Verification items for the finished model (mm, model axes). Face numbers are marked on the shaded views. A direction names the side the tool comes from. Round coordinates to 2 decimals unless told otherwise and drop trailing zeros. Loops run counter-clockwise (first coordinate to the right, second up) from the corner with the lowest first, then second, coordinate; pieces in that order, holes last. Notation, with made-up numbers: M -17.75,74.5 L -13.75,74.5 A18 cw -13.75,106.5 Z; hole C -31.75,1 d10. An arc over 180 degrees is marked long. Answer as CSV lines item,"result".
```python
from build123d import *

# Parameters (mm, degrees)
BOSS_EXTRUDE1_DEPTH = 4
BOSS_EXTRUDE2_DEPTH = 2.25
SKETCH3_R           = 7.925
CUT_EXTRUDE1_DEPTH  = 9.25
SKETCH4_R           = 2
CUT_EXTRUDE2_DEPTH  = 9.25
CUT_EXTRUDE3_DEPTH  = 3
FILLET1_R           = 2.36
CHAMFER1_SIZE       = 3.5
CHAMFER1_SIZE2      = 2.020725942
BOSS_EXTRUDE3_DEPTH = 4
FILLET2_R           = 2


with BuildPart() as part:
    # Sketch1 → Boss-Extrude1 (new body)
    with BuildSketch(Plane(origin=(0, 0, 0), x_dir=(1, 0, 0), z_dir=(0, 1, 0))):
        with BuildLine():
            Line((-13.29118379, 20.889836125), (-0.68999579, 20.889836125))
            Line((-0.68999579, 20.889836125), (-0.68999579, 24.09210312))
            Line((-0.68999579, 24.09210312), (-0.68999579, 26.09210312))
            Line((-0.68999579, 26.09210312), (12.01000421, 26.09210312))
            Line((12.01000421, 26.09210312), (12.01000421, 24.09210312))
            Line((12.01000421, 24.09210312), (12.01000421, -26.90789688))
            Line((12.01000421, -26.90789688), (12.01000421, -28.90789688))
            Line((12.01000421, -28.90789688), (-0.68999579, -28.90789688))
            Line((-0.68999579, -28.90789688), (-0.68999579, -26.90789688))
            Line((-0.68999579, -26.90789688), (-0.68999579, -23.705629885))
            Line((-0.68999579, -23.705629885), (-13.29118379, -23.705629885))
            ThreePointArc((-13.29118379, -23.705629885), (-35.588916795, -1.40789688), (-13.29118379, 20.889836125))
        make_face()
    extrude(amount=BOSS_EXTRUDE1_DEPTH)

    # Sketch2 → Boss-Extrude2 (add)
    with BuildSketch(Plane(origin=(0, 4, 0), x_dir=(1, 0, 0), z_dir=(0, 1, 0))):
        with BuildLine():
            Line((-0.68999579, 20.889836125), (-0.68999579, 16.987726462))
            ThreePointArc((-0.68999579, 16.987726462), (9.006549215, -1.40789688), (-0.68999579, -19.803520222))
            Line((-0.68999579, -19.803520222), (-0.68999579, -23.705629885))
            Line((-0.68999579, -23.705629885), (-13.29118379, -23.705629885))
            ThreePointArc((-13.29118379, -23.705629885), (-35.588916795, -1.40789688), (-13.29118379, 20.889836125))
            Line((-13.29118379, 20.889836125), (-0.68999579, 20.889836125))
        make_face()
    extrude(amount=BOSS_EXTRUDE2_DEPTH)

    # Sketch3 → Cut-Extrude1 (cut)
    with BuildSketch(Plane.XZ):
        with Locations(Location((-13.29118379, 1.40789688, 0), (0, 0, 270))):
            Circle(SKETCH3_R)
    extrude(amount=-CUT_EXTRUDE1_DEPTH, mode=Mode.SUBTRACT)

    # Sketch4 → Cut-Extrude2 (cut)
    with BuildSketch(Plane.XZ):
        with Locations(Location((3.31000421, -21.59210312, 0), (0, 0, 270))):
            Circle(SKETCH4_R)
        with Locations(Location((3.31000421, 24.40789688, 0), (0, 0, 270))):
            Circle(SKETCH4_R)
    extrude(amount=-CUT_EXTRUDE2_DEPTH, mode=Mode.SUBTRACT)

    # Sketch5 → Cut-Extrude3 (cut)
    with BuildSketch(Plane.XZ):
        with BuildLine():
            ThreePointArc((-20.901279021, -7.773174712), (-25.21618379, 1.40789688), (-20.901279021, 10.588968471))
            Line((-20.901279021, 10.588968471), (-24.18129969, 16.27013092))
            ThreePointArc((-24.18129969, 16.27013092), (-31.71618379, 1.40789688), (-24.18129969, -13.454337161))
            Line((-24.18129969, -13.454337161), (-20.901279021, -7.773174712))
        make_face()
        with BuildLine():
            Line((-20.717198075, 18.27013092), (-17.437177406, 12.588968471))
            ThreePointArc((-17.437177406, 12.588968471), (-7.32868379, 11.73524982), (-1.535094942, 3.40789688))
            Line((-1.535094942, 3.40789688), (5.024946397, 3.40789688))
            ThreePointArc((5.024946397, 3.40789688), (-4.07868379, 17.364414944), (-20.717198075, 18.27013092))
        make_face()
        with BuildLine():
            ThreePointArc((-1.535094942, -0.59210312), (-7.32868379, -8.91945606), (-17.437177406, -9.773174712))
            Line((-17.437177406, -9.773174712), (-20.717198075, -15.454337161))
            ThreePointArc((-20.717198075, -15.454337161), (-4.07868379, -14.548621185), (5.024946397, -0.59210312))
            Line((5.024946397, -0.59210312), (-1.535094942, -0.59210312))
        make_face()
    extrude(amount=-CUT_EXTRUDE3_DEPTH, mode=Mode.SUBTRACT)

    # Fillet1
    fillet1_edges = [part.edges().sort_by_distance(p)[0] for p in [
        (-20.901279021, 1.5, 10.588968471),
        (-20.901279021, 1.5, -7.773174712),
        (-24.18129969, 1.5, -13.454337161),
        (-24.18129969, 1.5, 16.27013092),
        (5.024946397, 1.5, 3.40789688),
        (-1.535094942, 1.5, 3.40789688),
        (-17.437177406, 1.5, 12.588968471),
        (-20.717198075, 1.5, 18.27013092),
        (-17.437177406, 1.5, -9.773174712),
        (-1.535094942, 1.5, -0.59210312),
        (5.024946397, 1.5, -0.59210312),
        (-20.717198075, 1.5, -15.454337161),
    ]]
    fillet(fillet1_edges, radius=FILLET1_R)

    # Chamfer1
    chamfer1_edges = [part.edges().sort_by_distance(p)[0] for p in [
        (12.01000421, 0, 1.40789688),
    ]]
    chamfer1_side = [part.faces().sort_by_distance(p)[0] for p in [
        (-3.714999267, 0, 17.994335016),
    ]]
    chamfer(chamfer1_edges, length=CHAMFER1_SIZE, length2=CHAMFER1_SIZE2, reference=chamfer1_side[0])

    # Sketch6 → Boss-Extrude3 (add)
    with BuildSketch(Plane.XZ):
        with BuildLine():
            Line((-0.68999579, -22.889836125), (-13.29118379, -22.889836125))
            ThreePointArc((-13.29118379, -22.889836125), (-37.588916795, 1.40789688), (-13.29118379, 25.705629885))
            Line((-13.29118379, 25.705629885), (-0.68999579, 25.705629885))
            Line((-0.68999579, 25.705629885), (-0.68999579, 23.705629885))
            Line((-0.68999579, 23.705629885), (-13.29118379, 23.705629885))
            ThreePointArc((-13.29118379, 23.705629885), (-35.588916795, 1.40789688), (-13.29118379, -20.889836125))
            Line((-13.29118379, -20.889836125), (-0.68999579, -20.889836125))
            Line((-0.68999579, -20.889836125), (-0.68999579, -22.889836125))
        make_face()
    extrude(amount=-BOSS_EXTRUDE3_DEPTH)

    # Fillet2
    fillet2_edges = [part.edges().sort_by_distance(p)[0] for p in [
        (-6.99058979, 0, 25.705629885),
        (-37.588916795, 0, 1.40789688),
        (-6.99058979, 0, -22.889836125),
    ]]
    fillet(fillet2_edges, radius=FILLET2_R)


solid = part.part
```
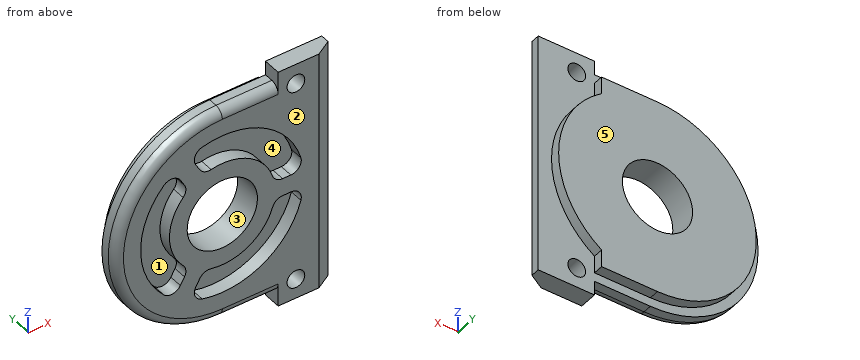
1) Set-up check for the marked faces 1 and 2: record each of +Z, -Z, +X, -X, +Y, -Y from which the full face is reachable in a straight line by a thin tool's end or side.
Here are the results:
face 1,"-Y"
face 2,"+Z, -Z, +X, -X, -Y"
2) Go/stop test with flat-tipped pins: pin 1 (0.6 mm diameter, centred on x = -9.5, y = 3.5, fed in from +Z); pin 2 (13 mm diameter, centred on x = -12, z = 12.5, fed in from -Y); pin 3 (2.5 mm diameter, centred on x = -8.5, y = 4.5, fed in from -Z); pin 4 (0.7 mm diameter, centred on y = 5, z = 22, fed in from +X). Record where each tip stops, or that it passes through.
Here are the results:
pin 1,"stops at z = 25.71"
pin 2,"stops at y = 0"
pin 3,"stops at z = -22.89"
pin 4,"stops at x = -0.69"
3) Section check A-A (y = 5.5). Record the cut outline in (x, z) (3 decimals), plus the area to 3 significant figures.
Here are the results:
outline,"M -13.291,-20.89 L -0.69,-20.89 L -0.69,-16.988 A22.298 ccw -0.69,19.804 L -0.69,23.706 L -13.291,23.706 A22.298 ccw Z; hole C -13.291,1.408 d15.85"
area,"1,400 mm^2"
4) Draft check along Z on the marked faces 3, 4 and 5. Enter one of: +Z half, -Z half, draft (parallel to the pull), parting line (faces both ways), or undercut.
Here are the results:
face 3,"undercut"
face 4,"undercut"
face 5,"draft"
5) Material ranges on probe 1 along Z at (x, y) = (-13, 5.5); probe 2 along Z at (x, y) = (-13, 2.75); probe 3 along X at (y, z) = (2.25, 0), recorded low to high.
Here are the results:
probe 1,"z = -20.89 to -6.51, 9.33 to 23.71"
probe 2,"z = -22.89 to -17.01, -10.51 to -6.51, 9.33 to 13.33, 19.83 to 25.71"
probe 3,"x = -37.55 to -31.66, -25.13 to -21.09, -5.49 to 12.01"
6) Section check C-C (y = 1). State how many separate pieces and enclosed holes the cut face has, plus the area to 3 significant figures.
Here are the results:
separate pieces,"1"
enclosed holes,"6"
area,"1,370 mm^2"
7) Section check B-B (x = 6). Record the cut outline in (y, z), plus the area to 3 significant figures.
Here are the results:
outline,"M 0,-26.09 L 4,-26.09 L 4,-9.77 L 6.25,-9.77 L 6.25,12.59 L 4,12.59 L 4,28.91 L 0,28.91 Z"
area,"270 mm^2"
